```python
from build123d import *

# Parameters (mm, degrees)
SKETCH1_W           = 83
SKETCH1_H           = 40
SKETCH1_R           = 2.05
SKETCH1_W_2         = 65
SKETCH1_H_2         = 31.325301204
BOSS_EXTRUDE1_DEPTH = 10


with BuildPart() as part:
    # Sketch1 → Boss-Extrude1 (new body)
    with BuildSketch(Plane(origin=(0, 0, 0), x_dir=(1, 0, 0), z_dir=(0, 1, 0))):
        Rectangle(SKETCH1_W, SKETCH1_H)
        with Locations(Location((-37.5, 8.5, 0), (0, 0, 270))):
            Circle(SKETCH1_R, mode=Mode.SUBTRACT)
        with Locations(Location((-37.5, -8.5, 0), (0, 0, 270))):
            Circle(SKETCH1_R, mode=Mode.SUBTRACT)
        with Locations(Location((37.5, -8.5, 0), (0, 0, 270))):
            Circle(SKETCH1_R, mode=Mode.SUBTRACT)
        with Locations(Location((37.5, 8.5, 0), (0, 0, 270))):
            Circle(SKETCH1_R, mode=Mode.SUBTRACT)
        Rectangle(SKETCH1_W_2, SKETCH1_H_2, mode=Mode.SUBTRACT)
    extrude(amount=BOSS_EXTRUDE1_DEPTH)


solid = part.part
```
Part model, mm, in its own coordinate system. A direction names the side the tool comes from. Give positions to 0.01 mm unless a question says otherwise; leave off trailing zeros. Order: outer loops, then holes, each group sorted by start corner. A loop starts at its lowest first (then second) coordinate and runs counter-clockwise, first axis right, second up. Notation, with made-up numbers: (87, 11.5) - (144, 11.5) arc R24 cw to (144, 30.5) - close; hole circle Ø9 at (13.25, 32). An arc over 180 degrees is marked (long way). Use one line per item in the form item = value.
Item 1: Which spindle directions (+Z, -Z, +X, -X, +Y, -Y) get a long thin tool onto all of the face, cutting with end or side? Do faces 4 (the face through (0, 5, 15.663)), 5 (the face through (-41.5, 5, 0)). Say none if no direction does.
Solution:
face_4 = +Y, -Y
face_5 = +Z, -Z, -X, +Y, -Y
Item 2: Pin check, flat tip, straight feed: pin 1 Ø3 at (x, z) = (0, 13) entering from +Y. Stop position of the tip, or through.
Solution:
pin_1 = through
Item 3: Slice it at B-B on z = 14. Give the cut face in (x, y).
Solution:
outline = (-41.5, 0) - (-32.5, 0) - (-32.5, 10) - (-41.5, 10) - close; (32.5, 0) - (41.5, 0) - (41.5, 10) - (32.5, 10) - close
Item 4: Probe probe 1 along X at (y, z) = (5, -8.5); probe 2 along Z at (x, y) = (2, 3.5); probe 3 along X at (y, z) = (2.25, 12). List the from-to ranges inside material, lowest first. Write a range as from..to.
Solution:
probe_1 = -41.5..-39.55, -35.45..-32.5, 32.5..35.45, 39.55..41.5
probe_2 = -20..-15.66, 15.66..20
probe_3 = -41.5..-32.5, 32.5..41.5
Item 5: Slice it at D-D on z = -8.5. Give the cut face in (x, y), and give its area (3 significant figures).
Solution:
outline = (-41.5, 0) - (-39.55, 0) - (-39.55, 10) - (-41.5, 10) - close; (-35.45, 0) - (-32.5, 0) - (-32.5, 10) - (-35.45, 10) - close; (32.5, 0) - (35.45, 0) - (35.45, 10) - (32.5, 10) - close; (39.55, 0) - (41.5, 0) - (41.5, 10) - (39.55, 10) - close
area = 98.0 mm2
Item 6: Slice it at C-C on x = -11. Give the cut face in (y, z).
Solution:
outline = (0, -20) - (10, -20) - (10, -15.66) - (0, -15.66) - close; (0, 15.66) - (10, 15.66) - (10, 20) - (0, 20) - close
Item 7: Slice it at A-A on x = -37.5. Give the cut face in (y, z).
Solution:
outline = (0, -20) - (10, -20) - (10, -10.55) - (0, -10.55) - close; (0, -6.45) - (10, -6.45) - (10, 6.45) - (0, 6.45) - close; (0, 10.55) - (10, 10.55) - (10, 20) - (0, 20) - close
Item 8: Two-plate mould, pull along Z, no slides. Class faces 1 (the face through (-1, 5, -20)), 2 (the face through (32.5, 5, 0)), 3 (the face through (41.5, 5, 0)): released by +Z, released by -Z, zero draft, split by the parting line, or undercut.
Solution:
face_1 = released by -Z
face_2 = undercut
face_3 = zero draft
